The drawing under review shows one solid part. Ordinate dimensions are in mm from its lowest x, y, z. A direction names the side the tool comes from. Give positions to 0.01 mm unless a question says otherwise; leave off trailing zeros. Loops run counter-clockwise (first coordinate to the right, second up) from the corner with the lowest first, then second, coordinate; pieces in that order, holes last. Notation, with made-up numbers: M 87,15.5 L 128,15.5 A36 cw 128,52.5 Z; hole C -21.75,-30 d9. An arc over 180 degrees is marked long. One line per item, written item: value. Start each with the question number.
Q1. For the marked faces 4 and 5, list the 3-axis set-ups (+Z, -Z, +X, -X, +Y, -Y) from which the entire face can be reached by the end or side of a thin tool; tool diameter is ignored.
Q2. We need section C-C on y = 17.5. Write out the cut boundary in (x, z).
Q3. We need section B-B on z = 1.23. Write out the cut boundary in (x, y) (3 decimals), plus the area to 3 significant figures.
Q4. We need section A-A on x = 3.2. Write out the cut boundary in (y, z) (3 decimals), plus the area to 3 significant figures.
Q5. To check wall thickness, follow line 1 along Z through (x, y) = (2.5, 8.75); line 2 along Y through (x, z) = (3.9, 2.9); line 3 along Y through (x, z) = (2.55, 0.95). State the ranges of each line that lie inside material, in increasing order. Write a range as from..to.
Q6. We need section D-D on x = 1.23. Write out the cut boundary in (y, z) (3 decimals).
Q7. Mouldability with a two-part tool opening along Z and no side actions: class the marked faces 1, 2 and 3 as released by +Z, released by -Z, zero draft, split by the parting line, or undercut.
Q8. For pin 1 (1.6 mm diameter, centred on y = 13, z = 2.5, fed in from +X), flat-tipped, find the tip position at first contact; note if it passes through.
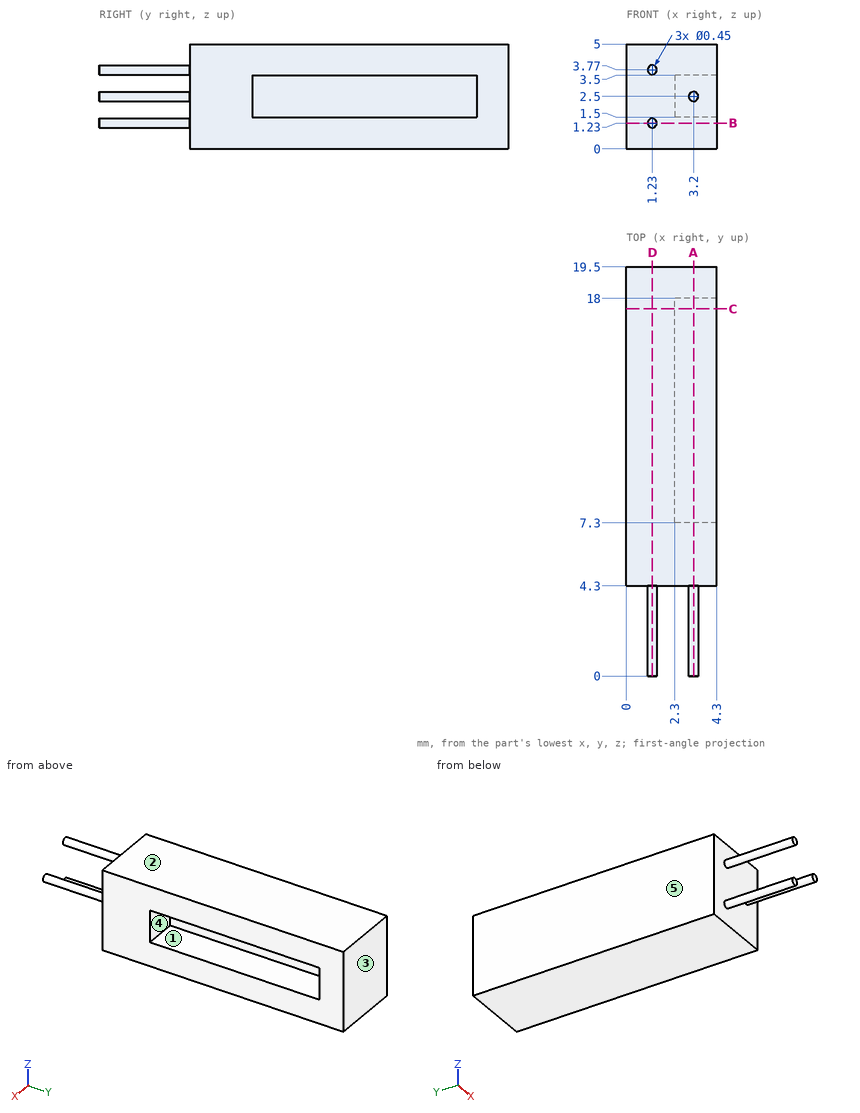
Solved:
1. face 4: +X
1. face 5: +Z, -Z, -X, +Y, -Y
2. outline: M 0,0 L 4.3,0 L 4.3,1.5 L 2.3,1.5 L 2.3,3.5 L 4.3,3.5 L 4.3,5 L 0,5 Z
3. outline: M 0,4.3 L 1.005,4.3 L 1.005,0 L 1.455,0 L 1.455,4.3 L 4.3,4.3 L 4.3,19.5 L 0,19.5 Z
3. area: 67.3 mm2
4. outline: M 0,2.275 L 4.3,2.275 L 4.3,0 L 19.5,0 L 19.5,5 L 4.3,5 L 4.3,2.725 L 0,2.725 Z; hole M 7.3,1.5 L 18,1.5 L 18,3.5 L 7.3,3.5 Z
4. area: 56.5 mm2
5. line 1: 0..1.5, 3.5..5
5. line 2: 4.3..7.3, 18..19.5
5. line 3: 4.3..19.5
6. outline: M 0,1.005 L 4.3,1.005 L 4.3,0 L 19.5,0 L 19.5,5 L 4.3,5 L 4.3,3.995 L 0,3.995 L 0,3.545 L 4.3,3.545 L 4.3,1.455 L 0,1.455 Z
7. face 1: undercut
7. face 2: released by +Z
7. face 3: zero draft
8. pin 1: x = 2.3
